Geometry check sheet. Reference: the model listing, model coordinates, mm. A direction names the side the tool comes from. Coordinates: 2 decimals unless noted, no trailing zeros. Write each loop counter-clockwise with the first axis right and the second up, starting at its lowest first coordinate (ties: lowest second). Pieces come first, ordered by that corner, then holes. Notation, with made-up numbers: (-17, -32) - (25, -32) arc R27 ccw to (25, -8) - close; hole circle Ø4 at (-7.5, 82.5). An arc over 180 degrees is marked (long way). Answer as a JSON object with one key per item and string values. Group by question number.
from build123d import *

# Parameters (mm, degrees)
BOSS_EXTRUDE1_DEPTH       = 43
SKETCH4_R                 = 10.207731482
SKETCH4_R_2               = 4.7
CUT_EXTRUDE3_DEPTH        = 11
CHAMFER3_SIZE             = 0.5
FILLET2_R                 = 0.5
F_1_0MM_DOWEL_HOLE1_D     = 6.35
F_1_0MM_DOWEL_HOLE1_DEPTH = 13
F_1_0MM_DOWEL_HOLE1_TIP   = 1.907732465
CHAMFER4_SIZE             = 0.5


with BuildPart() as part:
    # Sketch1 → Boss-Extrude1 (new body)
    with BuildSketch(Plane.XY):
        Polygon((0, 7.332348419), (-6.35, 3.666174209), (-6.35, -3.666174209), (0, -7.332348419), (6.35, -3.666174209), (6.35, 3.666174209), align=None)
    extrude(amount=BOSS_EXTRUDE1_DEPTH)

    # Sketch4 → Cut-Extrude3 (cut)
    with BuildSketch(Plane.XY.offset(43)):
        Circle(SKETCH4_R)
        Circle(SKETCH4_R_2, mode=Mode.SUBTRACT)
    extrude(amount=-CUT_EXTRUDE3_DEPTH, mode=Mode.SUBTRACT)

    # Chamfer3
    chamfer3_edges = [part.edges().sort_by_distance(p)[0] for p in [
        (-4.7, 0, 43),
    ]]
    chamfer(chamfer3_edges, length=CHAMFER3_SIZE)

    # Fillet2
    fillet2_edges = [part.edges().sort_by_distance(p)[0] for p in [
        (-4.7, 0, 32),
    ]]
    fillet(fillet2_edges, radius=FILLET2_R)

    # Ø1.0mm Dowel Hole1
    with Locations(Plane(origin=(0, 0, 0), x_dir=(-1, 0, 0), z_dir=(0, 0, -1))):
        with Locations((0, 0)):
            Hole(F_1_0MM_DOWEL_HOLE1_D / 2, depth=F_1_0MM_DOWEL_HOLE1_DEPTH)
            with Locations((0, 0, -(F_1_0MM_DOWEL_HOLE1_DEPTH + F_1_0MM_DOWEL_HOLE1_TIP / 2))):  # 118° drill point
                Cone(0, F_1_0MM_DOWEL_HOLE1_D / 2, F_1_0MM_DOWEL_HOLE1_TIP, mode=Mode.SUBTRACT)

    # Chamfer4
    chamfer4_edges = [part.edges().sort_by_distance(p)[0] for p in [
        (-3.175, 0, 0),
    ]]
    chamfer(chamfer4_edges, length=CHAMFER4_SIZE)


solid = part.part
(1) Draft check along Y on faces 3 (the face through (0, 0, 43)), 4 (the face through (-3.219, -5.474, 15.776)), 5 (the face through (0.1, -0.5, 14.6)), 6 (the face through (-0.69, -3.1, 6.84)). Enter one of: +Y half, -Y half, draft (parallel to the pull), parting line (faces both ways), or undercut.
(2) Gauge pin test, flat ends, axial feed: pin 1 (3 mm diameter, centred on y = 6, z = 27.5, fed in from +X); pin 2 (6 mm diameter, centred on x = 4, z = 8.5, fed in from -Y) (3 decimals); pin 3 (6 mm diameter, centred on x = 1.5, z = 11.5, fed in from -Y). Record the tip position at first contact, or that the pin passes through.
(3) Section check A-A (z = 6.5). Record the cut outline in (x, y) (3 decimals).
(4) Set-up check for faces 1 (the face through (-4.3, -3.2, 32)), 2 (the face through (3.219, 5.474, 15.776)): record each of +Z, -Z, +X, -X, +Y, -Y from which the full face is reachable in a straight line by a thin tool's end or side.
(5) Section check B-B (z = 19.5). Record the cut outline in (x, y), and give its area (3 significant figures).
(6) Material ranges on L1, parallel to Y at x = 0, z = 5 (3 decimals); L2, parallel to X at y = 0, z = 4.5 (3 decimals); L3, parallel to Z at x = -1.5, y = 5.75, recorded low to high. Write a range as [from, to].
Conclusion:
{
 "1": {"face 3": "draft", "face 4": "-Y half", "face 5": "undercut", "face 6": "undercut"},
 "2": {"pin 1": "stops at x = 4.91", "pin 2": "stops at y = -6.755", "pin 3": "stops at y = -7.33"},
 "3": {"outline": "(-6.35, -3.666) - (0, -7.332) - (6.35, -3.666) - (6.35, 3.666) - (0, 7.332) - (-6.35, 3.666) - close; hole circle Ø6.35 at (0, 0)"},
 "4": {"face 1": "+Z", "face 2": "+Z, -Z, +X, +Y"},
 "5": {"outline": "(-6.35, -3.67) - (0, -7.33) - (6.35, -3.67) - (6.35, 3.67) - (0, 7.33) - (-6.35, 3.67) - close", "area": "140 mm^2"},
 "6": {"L1": "y = [-7.332, -3.175], [3.175, 7.332]", "L2": "x = [-6.35, -3.175], [3.175, 6.35]", "L3": "z = [0, 32]"}
}
